from build123d import *

# Parameters (mm, degrees)
PAD_DEPTH    = 2
POCKET_DEPTH = 1
FILLET_R     = 3
FILLET001_R  = 4.5


with BuildPart() as part:
    # Sketch → Pad (new body)
    with BuildSketch(Plane.XY):
        with BuildLine():
            ThreePointArc((0, 6), (39, 0), (78, 6))
            Line((78, 133), (78, 6))
            Line((0, 133), (78, 133))
            Line((0, 6), (0, 133))
        make_face()
    extrude(amount=PAD_DEPTH)

    # Sketch001 (on Face6 of Pad) → Pocket (cut)
    with BuildSketch(Plane.XY.offset(2)):
        with BuildLine():
            ThreePointArc((4.5, 68.5), (39, 66.5), (73.5, 68.5))
            Line((73.5, 127.5), (73.5, 68.5))
            Line((4.5, 127.5), (73.5, 127.5))
            Line((4.5, 68.5), (4.5, 127.5))
        make_face()
    extrude(amount=-POCKET_DEPTH, mode=Mode.SUBTRACT)

    # Fillet
    fillet_edges = [part.edges().sort_by_distance(p)[0] for p in [
        (73.5, 68.5, 1.5),
        (73.5, 127.5, 1.5),
        (4.5, 127.5, 1.5),
        (4.5, 68.5, 1.5),
    ]]
    fillet(fillet_edges, radius=FILLET_R)

    # Fillet001
    fillet001_edges = [part.edges().sort_by_distance(p)[0] for p in [
        (78, 6, 1),
        (78, 133, 1),
        (0, 6, 1),
        (0, 133, 1),
    ]]
    fillet(fillet001_edges, radius=FILLET001_R)


solid = part.part
The listing builds one solid part. Answer for the finished solid, in the listing's coordinates (mm). A direction names the side the tool comes from. Coordinates: 2 decimals unless noted, no trailing zeros. Write each loop counter-clockwise with the first axis right and the second up, starting at its lowest first coordinate (ties: lowest second). Pieces come first, ordered by that corner, then holes. Notation, with made-up numbers: M 86,85.5 L 129,85.5 A33 ccw 129,120.5 Z; hole C 35,28 d11. An arc over 180 degrees is marked long. Use one line per item in the form item = value.
Item 1: Find the intervals of material crossed by probe 1 along X at (y, z) = (115, 1.55); probe 2 along Z at (x, y) = (57, 69.5); probe 3 along Y at (x, z) = (24.5, 1.95), in increasing order.
Model answer:
probe_1 = 0 to 4.5, 73.5 to 78
probe_2 = 0 to 1
probe_3 = 0.81 to 66.85, 127.5 to 133
Item 2: For faces 5 (the face through (38, 67, 0)), 6 (the face through (5.289, 69.156, 1.493)), determine the directions among +Z, -Z, +X, -X, +Y, -Y from which every point of the face is accessible in a straight line to the end or side of a thin tool.
Model answer:
face_5 = -Z, +X, -X, +Y, -Y
face_6 = +Z
Item 3: Find section C-C, the plane x = 17.5. Give the vertices of the cut face in (y, z).
Model answer:
outline = M 1.79,0 L 133,0 L 133,2 L 127.5,2 L 127.5,1 L 67.28,1 L 67.28,2 L 1.79,2 Z
Item 4: Find section B-B, the plane y = 90. Give the vertices of the cut face in (x, z).
Model answer:
outline = M 0,0 L 78,0 L 78,2 L 73.5,2 L 73.5,1 L 4.5,1 L 4.5,2 L 0,2 Z
Item 5: Given P1, Ø8, axis at x = 34.5, y = 75, coming from the +Z side; P2, Ø0.5, axis at x = 32.5, z = 1.5, coming from the -Y side, each flat-ended and moving along its own axis, determine where each tip first touches the part or whether it passes through.
Model answer:
P1 = 1
P2 = 0.15
Item 6: The mould has two halves that part along X. Classify faces 1 (the face through (38.5, 0, 1)), 2 (the face through (72.64, 126.6, 1.49)), 3 (the face through (1.283, 131.647, 1.014)), 4 (the face through (5.4, 126.64, 1.49)): released by +X, released by -X, zero draft, split by the parting line, or undercut.
Model answer:
face_1 = split by the parting line
face_2 = undercut
face_3 = released by -X
face_4 = undercut
